The model under review builds one solid part; all positions refer to its coordinate system, in mm. A direction names the side the tool comes from. Round coordinates to 2 decimals unless told otherwise and drop trailing zeros. Order: outer loops, then holes, each group sorted by start corner. A loop starts at its lowest first (then second) coordinate and runs counter-clockwise, first axis right, second up. Notation, with made-up numbers: (43.25, 4.25) -> (66.25, 4.25) arc R16 cw to (66.25, 30.25) -> close; hole circle Ø10 at (-5, 9.25). An arc over 180 degrees is marked (long way). Use a Markdown table: item, result. Add a question column.
```python
from build123d import *

# Parameters (mm, degrees)
SKETCH_1_R          = 3
EXTRUDE_1_DEPTH     = 10
SKETCH_2_R          = 1
CUT_EXTRUDE_1_DEPTH = 5
CUT_EXTRUDE_START   = 10
SKETCH_3_R          = 1.5
CUT_EXTRUDE_2_DEPTH = 5
CHAMFER_1_SIZE      = 0.2
CHAMFER_2_SIZE      = 0.1


with BuildPart() as part:
    # 草图1 → 凸台-拉伸1 (new body)
    with BuildSketch(Plane(origin=(0, 0, 0), x_dir=(1, 0, 0), z_dir=(0, 1, 0))):
        with Locations(Location((0, 0, 0), (0, 0, 270))):
            Circle(SKETCH_1_R)
    extrude(amount=EXTRUDE_1_DEPTH)

    # 草图2 → 切除-拉伸1 (cut)
    with BuildSketch(Plane(origin=(0, 0, 0), x_dir=(1, 0, 0), z_dir=(0, 1, 0))):
        with Locations(Location((0, 0, 0), (0, 0, 270))):
            Circle(SKETCH_2_R)
    extrude(amount=CUT_EXTRUDE_1_DEPTH, mode=Mode.SUBTRACT)

    # 草图3 → 切除-拉伸2 (cut)
    with BuildSketch(Plane(origin=(0, 0, 0), x_dir=(1, 0, 0), z_dir=(0, 1, 0)).offset(CUT_EXTRUDE_START)):
        with Locations(Location((0, 0, 0), (0, 0, 270))):
            Circle(SKETCH_3_R)
    extrude(amount=-CUT_EXTRUDE_2_DEPTH, mode=Mode.SUBTRACT)

    # 倒角1
    chamfer_1_edges = [part.edges().sort_by_distance(p)[0] for p in [
        (0, 0, -3),
        (0, 10, -3),
    ]]
    chamfer(chamfer_1_edges, length=CHAMFER_1_SIZE)

    # 倒角2
    chamfer_2_edges = [part.edges().sort_by_distance(p)[0] for p in [
        (0, 10, -1.5),
        (0, 0, -1),
    ]]
    chamfer(chamfer_2_edges, length=CHAMFER_2_SIZE)


solid = part.part
```
Q1. Add section D-D (y = 6.75). Write out the cut boundary in (x, z), then the cut area to 3 significant figures.
Q2. Add section B-B (z = 0). Write out the cut boundary in (x, y), then the cut area to 3 significant figures.
Q3. Machinability: for faces 4 (the cylindrical face through (0.45, 7.48, 1.43)), 5 (the flat face through (-1, 0, 1)), which of the approach directions +Z, -Z, +X, -X, +Y, -Y give a long, thin tool a straight path to every point of the face, cutting with its end or side? Answer none if there is none.
Q4. Mouldability with a two-part tool opening along Z and no side actions: class faces 1 (the cylindrical face through (-1, 3, 0)), 2 (the flat face through (-2, 10, 0)), 3 (the cylindrical face through (0.9, 4.93, 2.86)) as pulls with the +Z half, pulls with the -Z half, needs draft (parallel to the pull), parting line crosses it, or undercut.
Q5. Add section C-C (y = 2.5). Write out the cut boundary in (x, z).
Q6. Insertion check: pin 1 (1 mm diameter, centred on y = 1.5, z = -2, fed in from -X); pin 2 (2 mm diameter, centred on y = 7.5, z = -2, fed in from -X); pin 3 (1 mm diameter, centred on x = -1.5, y = 6, fed in from -Z). Each pin has a flat end and moves straight along its axis. Give the tip position at first contact, or say it passes through.
Q7. Wall thickness on line 1 (X direction, y = 1.2, z = 0); line 2 (X direction, y = 8.5, z = 1.2); line 3 (Z direction, x = 0.65, y = 2): over which ranges is each line inside the solid? List them lowest first. Write a range as [from, to].
Q8. Add section A-A (x = 0). Write out the cut boundary in (y, z), then the cut area to 3 significant figures.
Report:
| question | item | result |
|---|---|---|
| 1 | outline | circle Ø6 at (0, 0); hole circle Ø3 at (0, 0) |
| 1 | area | 21.2 mm² |
| 2 | outline | (-3, 0.2) -> (-2.8, 0) -> (-1.1, 0) -> (-1, 0.1) -> (-1, 5) -> (-1.5, 5) -> (-1.5, 9.9) -> (-1.6, 10) -> (-2.8, 10) -> (-3, 9.8) -> close; (1, 0.1) -> (1.1, 0) -> (2.8, 0) -> (3, 0.2) -> (3, 9.8) -> (2.8, 10) -> (1.6, 10) -> (1.5, 9.9) -> (1.5, 5) -> (1, 5) -> close |
| 2 | area | 34.9 mm² |
| 3 | face 4 | +Y |
| 3 | face 5 | +Z, -Z, +X, -X, -Y |
| 4 | face 1 | undercut |
| 4 | face 2 | needs draft |
| 4 | face 3 | parting line crosses it |
| 5 | outline | circle Ø6 at (0, 0); hole circle Ø2 at (0, 0) |
| 6 | pin 1 | stops at x = -2.6 |
| 6 | pin 2 | stops at x = -2.83 |
| 6 | pin 3 | stops at z = -2.83 |
| 7 | line 1 | x = [-3, -1], [1, 3] |
| 7 | line 2 | x = [-2.75, -0.9], [0.9, 2.75] |
| 7 | line 3 | z = [-2.93, -0.76], [0.76, 2.93] |
| 8 | outline | (0, -2.8) -> (0.2, -3) -> (9.8, -3) -> (10, -2.8) -> (10, -1.6) -> (9.9, -1.5) -> (5, -1.5) -> (5, -1) -> (0.1, -1) -> (0, -1.1) -> close; (0, 1.1) -> (0.1, 1) -> (5, 1) -> (5, 1.5) -> (9.9, 1.5) -> (10, 1.6) -> (10, 2.8) -> (9.8, 3) -> (0.2, 3) -> (0, 2.8) -> close |
| 8 | area | 34.9 mm² |
